Autodesk Inventor part; units mm, degrees
ref_plane "YZ Plane" through (0, 0, 0) normal (1, 0, 0) x (0, 1, 0)
ref_plane "XZ Plane" through (0, 0, 0) normal (0, 1, 0) x (-1, 0, 0)
ref_plane "XY Plane" through (0, 0, 0) normal (0, 0, 1) x (1, 0, 0)
sketch "Sketch1" plane through (0, 0, 0) normal (0, 0, 1) x (1, 0, 0)
  circle A0 centre (0, 0) radius 7.94 construction
  circle A1 centre (0, 0) radius 8.44
  point P0 (0, 0)
  dimension "d5" = 0.5
extrude "Extrusion1" add sketch "Sketch1" along normal blind 10 and the other way blind 20
sketch "Sketch2" plane through (0, 0, 0) normal (1, 0, 0) x (0, 1, 0)
  line L0 (-8.44, -20) -> (8.44, -20) construction
  line L1 (8.44, 10) -> (-8.44, 10) construction
  line L2 (8.44, 10) -> (8.44, -20)
  line L3 (8.44, 10) -> (6.44, -20)
  line L4 (8.44, -20) -> (6.44, -20)
  line L5 (0, -26) -> (0, 16)
  point P0 (0, 0)
  dimension "d6" = 2
revolve "Revolution1" cut sketch "Sketch2" angle 360 about axis through (0, 0, 10) along (0, 0, 1)
sketch "Sketch3" plane through (0, 0, -20) normal (0, 0, -1) x (-1, 0, 0)
  circle A0 centre (0, 0) radius 6.44 construction
  circle A1 centre (0, 0) radius 3.94
  dimension "d8" = 2.5
extrude "Extrusion2" cut sketch "Sketch3" against normal through all
sketch "Sketch4" plane through (0, 0, 10) normal (0, 0, 1) x (1, 0, 0)
  circle A0 centre (0, 0) radius 3.94
  circle A1 centre (0, 0) radius 8.44
extrude "Extrusion3" add sketch "Sketch4" along normal blind 15
properties part number "Vented_plug"
CAD build for the part. Positions are in the model's coordinates, mm. Round coordinates to 2 decimals unless told otherwise and drop trailing zeros. Loops run counter-clockwise (first coordinate to the right, second up) from the corner with the lowest first, then second, coordinate; pieces in that order, holes last.
(1) Cut at C-C (z = -2.5). Give the cut face in (x, y), plus the area to 3 significant figures.
(2) Wall check: line 1 along Y through (x, z) = (0, 11.5); line 2 along X through (y, z) = (0, -2); line 3 along X through (y, z) = (0, 7). Give the ranges that are in metal, low to high.
(3) Two-plate mould, pull along X, no slides. Class faces 1 (the conical face through (6.613, 3.44, -4.79)), 2 (the flat face through (4, -2, 25)), 3 (the cylindrical face through (-0.26, 3.93, 2.18)): +X half, -X half, draft (parallel to the pull), parting line (faces both ways), or undercut.
(4) Cut at D-D (z = -15). Give the cut face in (x, y).
(5) Drop flat-ended pins along their axis: pin 1 (8 mm diameter, centred on y = 2, z = 15, fed in from +X); pin 2 (1.5 mm diameter, centred on x = -1.5, z = -13.5, fed in from +Y); pin 3 (8 mm diameter, centred on x = -3, z = -14, fed in from -Y); pin 4 (5 mm diameter, centred on y = -6, z = 5, fed in from -X). Give the stop position or say it passes through.
(6) Cut at A-A (x = 0). Give the cut face in (y, z), plus the area to 3 significant figures.
Findings below:
1. outline: circle Ø15.21 at (0, 0); hole circle Ø7.88 at (0, 0)
1. area: 133 mm2
2. line 1: y = -8.44 to -3.94, 3.94 to 8.44
2. line 2: x = -7.64 to -3.94, 3.94 to 7.64
2. line 3: x = -8.24 to -3.94, 3.94 to 8.24
3. face 1: parting line
3. face 2: draft
3. face 3: undercut
4. outline: circle Ø13.55 at (0, 0); hole circle Ø7.88 at (0, 0)
5. pin 1: stops at x = 8.44
5. pin 2: stops at y = 6.85
5. pin 3: stops at y = -7.03
5. pin 4: stops at x = -7.33
6. outline: (-8.44, 10) - (-6.44, -20) - (-3.94, -20) - (-3.94, 25) - (-8.44, 25) - close; (3.94, -20) - (6.44, -20) - (8.44, 10) - (8.44, 25) - (3.94, 25) - close
6. area: 345 mm2
